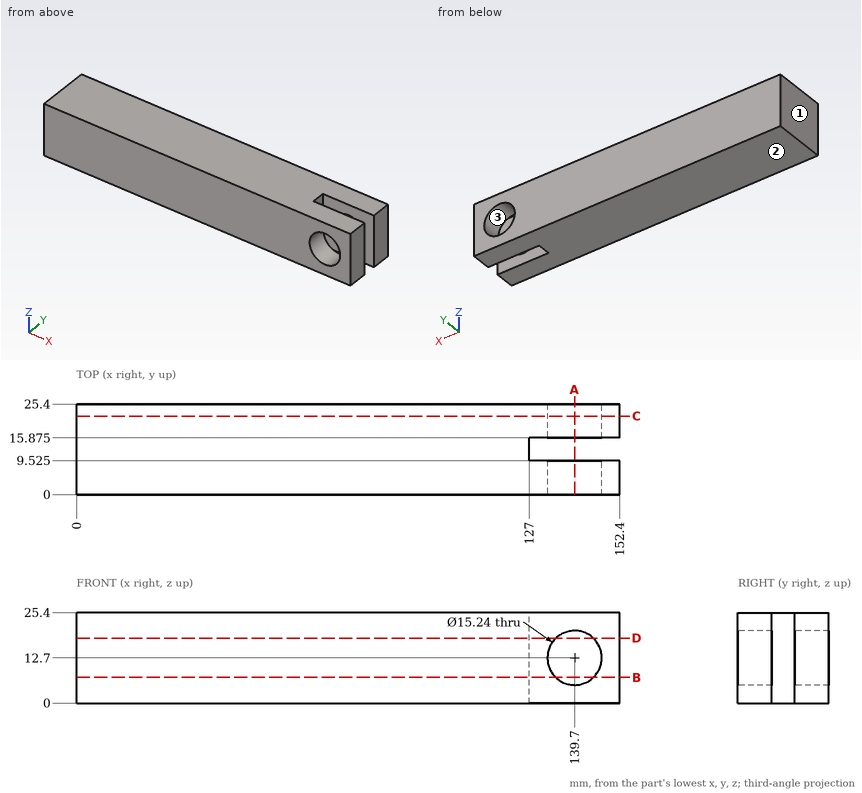
Verification items for this drawing (mm, ordinates from the low corner). Give positions to 0.01 mm unless a question says otherwise; leave off trailing zeros. Write each loop counter-clockwise with the first axis right and the second up, starting at its lowest first coordinate (ties: lowest second). Pieces come first, ordered by that corner, then holes.
1) Gauge pin test, flat ends, axial feed: pin 1 (1.5 mm diameter, centred on x = 67, y = 19.5, fed in from -Z); pin 2 (13.5 mm diameter, centred on x = 139.7, z = 12.7, fed in from +Y); pin 3 (1.9 mm diameter, centred on y = 13.5, z = 7, fed in from +X). Record the tip position at first contact, or that the pin passes through.
2) Section check C-C, the plane y = 22. Record the boundary of the cut face in (x, z).
3) Material ranges on L1, parallel to Z at x = 139.7, y = 3.75; L2, parallel to Y at x = 134, z = 24 (3 decimals); L3, parallel to X at y = 14.5, z = 11.5, recorded low to high.
4) Section check D-D, the plane z = 18.25. Record the boundary of the cut face in (x, y) (3 decimals).
5) Section check A-A, the plane x = 139.7. Record the boundary of the cut face in (y, z) (3 decimals), and give its area (3 significant figures).
6) Section check B-B, the plane z = 7.25. Record the boundary of the cut face in (x, y) (3 decimals), and give its area (3 significant figures).
7) Release check for a two-part mould opening along X. For the marked faces 1, 2 and 3 record: pulls with the +X half, pulls with the -X half, needs draft (parallel to the pull), parting line crosses it, or undercut.
Computed:
1. pin 1: stops at z = 0
1. pin 2: passes through
1. pin 3: stops at x = 127
2. outline: (0, 0) - (152.4, 0) - (152.4, 25.4) - (0, 25.4) - close; hole circle Ø15.24 at (139.7, 12.7)
3. L1: z = 0 to 5.08, 20.32 to 25.4
3. L2: y = 0 to 9.525, 15.875 to 25.4
3. L3: x = 0 to 127
4. outline: (0, 0) - (134.479, 0) - (134.479, 9.525) - (127, 9.525) - (127, 15.875) - (134.479, 15.875) - (134.479, 25.4) - (0, 25.4) - close; (144.921, 0) - (152.4, 0) - (152.4, 9.525) - (144.921, 9.525) - close; (144.921, 15.875) - (152.4, 15.875) - (152.4, 25.4) - (144.921, 25.4) - close
5. outline: (0, 0) - (9.525, 0) - (9.525, 5.08) - (0, 5.08) - close; (0, 20.32) - (9.525, 20.32) - (9.525, 25.4) - (0, 25.4) - close; (15.875, 0) - (25.4, 0) - (25.4, 5.08) - (15.875, 5.08) - close; (15.875, 20.32) - (25.4, 20.32) - (25.4, 25.4) - (15.875, 25.4) - close
5. area: 194 mm2
6. outline: (0, 0) - (134.374, 0) - (134.374, 9.525) - (127, 9.525) - (127, 15.875) - (134.374, 15.875) - (134.374, 25.4) - (0, 25.4) - close; (145.026, 0) - (152.4, 0) - (152.4, 9.525) - (145.026, 9.525) - close; (145.026, 15.875) - (152.4, 15.875) - (152.4, 25.4) - (145.026, 25.4) - close
6. area: 3,510 mm2
7. face 1: pulls with the -X half
7. face 2: needs draft
7. face 3: undercut
